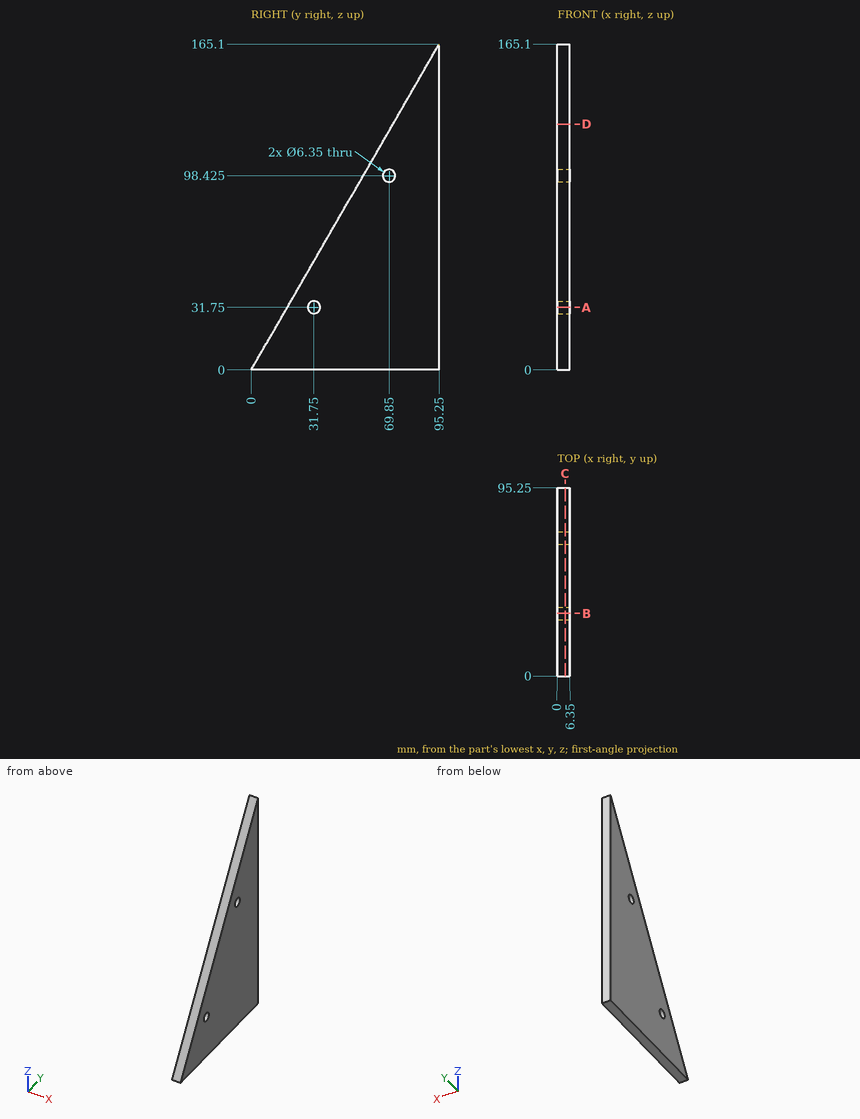
The drawing under review shows one solid part. Ordinate dimensions are in mm from its lowest x, y, z. Give positions to 0.01 mm unless a question says otherwise; leave off trailing zeros. Write each loop counter-clockwise with the first axis right and the second up, starting at its lowest first coordinate (ties: lowest second). Pieces come first, ordered by that corner, then holes. Notation, with made-up numbers: (9, 61) -> (64, 61) arc R4 cw to (64, 65) -> close; hole circle Ø3 at (-31.75, -20). An arc over 180 degrees is marked (long way). Use CSV: the item, a comma, the result in double quotes.
Q1. Take a section at B-B, the plane y = 31.75. Write out the cut boundary in (x, z) (3 decimals).
Conclusion:
outline,"(0, 0) -> (6.35, 0) -> (6.35, 28.575) -> (0, 28.575) -> close; (0, 34.925) -> (6.35, 34.925) -> (6.35, 55.033) -> (0, 55.033) -> close"
Q2. Take a section at D-D, the plane z = 124.5. Write out the cut boundary in (x, y).
Conclusion:
outline,"(0, 71.83) -> (6.35, 71.83) -> (6.35, 95.25) -> (0, 95.25) -> close"
Q3. To check wall thickness, follow probe 1 along Z at (x, y) = (1.5, 31.75) (3 decimals); probe 2 along Z at (x, y) = (3.25, 69.85); probe 3 along Y at (x, z) = (1, 100). State the ranges of each line that lie inside material, in increasing order. Write a range as [from, to].
Conclusion:
probe 1,"[0, 28.575], [34.925, 55.033]"
probe 2,"[0, 95.25], [101.6, 121.07]"
probe 3,"[57.69, 67.09], [72.61, 95.25]"
Q4. Take a section at A-A, the plane z = 31.75. Write out the cut boundary in (x, y) (3 decimals).
Conclusion:
outline,"(0, 18.317) -> (6.35, 18.317) -> (6.35, 28.575) -> (0, 28.575) -> close; (0, 34.925) -> (6.35, 34.925) -> (6.35, 95.25) -> (0, 95.25) -> close"
Q5. For P1, Ø1, axis at x = 2.5, y = 75, coming from the -Z side; P2, Ø1.5, axis at x = 5, y = 50, coming from the +Z side; P3, Ø4, axis at y = 31.75, z = 31.75, coming from the +X side, all flat-tipped, find the tip position at first contact; note any pin that passes through.
Conclusion:
P1,"z = 0"
P2,"z = 87.97"
P3,"through"
Q6. Take a section at C-C, the plane x = 4. Write out the cut boundary in (y, z) (3 decimals).
Conclusion:
outline,"(0, 0) -> (95.25, 0) -> (95.25, 165.1) -> close; hole circle Ø6.35 at (31.75, 31.75); hole circle Ø6.35 at (69.85, 98.425)"
